Could you check a few things on this model? Use its own coordinates, in mm. Face numbers are marked on the shaded views. A direction names the side the tool comes from. Round coordinates to 2 decimals unless told otherwise and drop trailing zeros. Write each loop counter-clockwise with the first axis right and the second up, starting at its lowest first coordinate (ties: lowest second). Pieces come first, ordered by that corner, then holes. Notation, with made-up numbers: (-38.75, 12.5) - (-7.75, 12.5) arc R5 ccw to (-7.75, 20.5) - close; hole circle Ø6 at (10, 6). An arc over 180 degrees is marked (long way). Put each result on its own line as item: value.
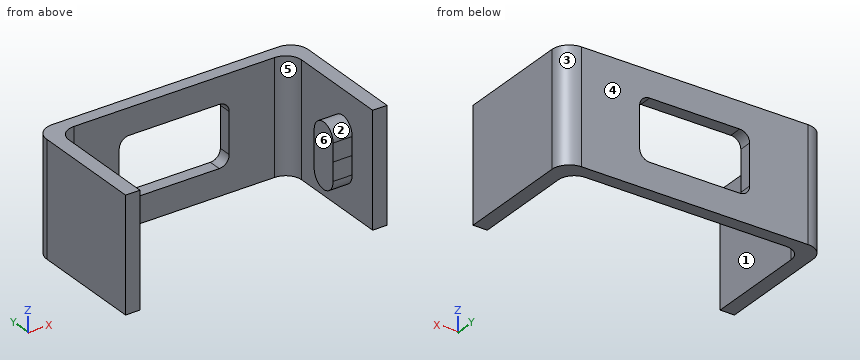
from build123d import *

# Parameters (mm, degrees)
F1_DEPTH = 9.017
F3_DEPTH = 10.288
F5_DEPTH = 2.54
F7_DEPTH = 9.017
F9_DEPTH = 25.4


with BuildPart() as f1:
    # F0 (on Top) → F1 (new body)
    with BuildSketch(Plane.XY):
        with BuildLine():
            Line((0, 9.017), (0, 0))
            Line((0, 0), (1.016, 0))
            Line((1.016, 0), (1.016, 8.128))
            ThreePointArc((1.016, 8.128), (1.387974, 9.026026), (2.286, 9.398))
            Line((2.286, 9.398), (18.288, 9.398))
            ThreePointArc((18.288, 9.398), (19.186026, 9.026026), (19.558, 8.128))
            Line((19.558, 8.128), (19.558, 0))
            Line((19.558, 0), (20.574, 0))
            Line((20.574, 0), (20.574, 9.017))
            ThreePointArc((20.574, 9.017), (20.202026, 9.915026), (19.304, 10.287))
            Line((19.304, 10.287), (1.27, 10.287))
            ThreePointArc((1.27, 10.287), (0.371974, 9.915026), (0, 9.017))
        make_face()
    extrude(amount=F1_DEPTH)

    # F2 (on face) → F3 (cut, through all)
    with BuildSketch(Plane(origin=(0, 10.287, 0), x_dir=(-1, 0, 0), z_dir=(0, 1, 0))):
        with BuildLine():
            Line((-13.87475, 2.0955), (-6.69925, 2.0955))
            ThreePointArc((-6.69925, 2.0955), (-6.137984, 2.327984), (-5.9055, 2.88925))
            Line((-5.9055, 2.88925), (-5.9055, 6.12775))
            ThreePointArc((-5.9055, 6.12775), (-6.137984, 6.689016), (-6.69925, 6.9215))
            Line((-6.69925, 6.9215), (-13.87475, 6.9215))
            ThreePointArc((-13.87475, 6.9215), (-14.436016, 6.689016), (-14.6685, 6.12775))
            Line((-14.6685, 6.12775), (-14.6685, 2.88925))
            ThreePointArc((-14.6685, 2.88925), (-14.436016, 2.327984), (-13.87475, 2.0955))
        make_face()
    extrude(amount=-F3_DEPTH, mode=Mode.SUBTRACT)

    # F4 (on face) → F5 (join)
    with BuildSketch(Plane.YZ.offset(20.574)):
        with BuildLine():
            Line((4.503683, 2.984615), (4.525844, 4.5085))
            Line((4.525844, 4.5085), (4.503683, 6.032385))
            ThreePointArc((4.503683, 6.032385), (3.385713, 7.047766), (2.345612, 5.952756))
            Line((2.345612, 5.952756), (2.366616, 4.5085))
            Line((2.366616, 4.5085), (2.345612, 3.064244))
            ThreePointArc((2.345612, 3.064244), (3.385713, 1.969234), (4.503683, 2.984615))
        make_face()
    extrude(amount=-F5_DEPTH)

    # F6 (on face) → F7 (join, through all)
    with BuildSketch(Plane(origin=(0, 0, 0), x_dir=(1, 0, 0), z_dir=(0, 0, -1))):
        with BuildLine():
            Line((20.574, 0), (20.574, -9.017))
            ThreePointArc((20.574, -9.017), (20.202026, -9.915026), (19.304, -10.287))
            Line((19.304, -10.287), (1.27, -10.287))
            ThreePointArc((1.27, -10.287), (0.371974, -9.915026), (0, -9.017))
            Line((0, -9.017), (0, 0))
            Line((0, 0), (-0.127, 0))
            Line((-0.127, 0), (-0.127, -9.017))
            ThreePointArc((-0.127, -9.017), (0.282172, -10.004828), (1.27, -10.414))
            Line((1.27, -10.414), (19.304, -10.414))
            ThreePointArc((19.304, -10.414), (20.291828, -10.004828), (20.701, -9.017))
            Line((20.701, -9.017), (20.701, 0))
            Line((20.701, 0), (20.574, 0))
        make_face()
    extrude(amount=-F7_DEPTH)

    # F8 (on face) → F9 (cut)
    with BuildSketch(Plane.XZ.offset(-10.287)):
        with BuildLine():
            ThreePointArc((5.9055, 2.88925), (6.137984, 2.327984), (6.69925, 2.0955))
            Line((6.69925, 2.0955), (13.87475, 2.0955))
            ThreePointArc((13.87475, 2.0955), (14.436016, 2.327984), (14.6685, 2.88925))
            Line((14.6685, 2.88925), (14.6685, 6.12775))
            ThreePointArc((14.6685, 6.12775), (14.436016, 6.689016), (13.87475, 6.9215))
            Line((13.87475, 6.9215), (6.69925, 6.9215))
            ThreePointArc((6.69925, 6.9215), (6.137984, 6.689016), (5.9055, 6.12775))
            Line((5.9055, 6.12775), (5.9055, 2.88925))
        make_face()
    extrude(amount=-F9_DEPTH, mode=Mode.SUBTRACT)


solid = f1.part
(1) If we mould it in two halves opening along Y, with no side actions, what happens to the marked faces 1, 2 and 3? For each: pulls with the +Y half, pulls with the -Y half, needs draft (parallel to the pull), parting line crosses it, or undercut.
Values found:
face 1: needs draft
face 2: undercut
face 3: pulls with the +Y half
(2) Imagine slicing it at B-B, the plane x = 13.5. List the corners of the cut face in (y, z) for me.
Values found:
outline: (9.4, 0) - (10.41, 0) - (10.41, 2.1) - (9.4, 2.1) - close; (9.4, 6.92) - (10.41, 6.92) - (10.41, 9.02) - (9.4, 9.02) - close
(3) Imagine slicing it at C-C, the plane z = 5.5. List the corners of the cut face in (x, y) for me, then the cut area to 3 significant figures.
Values found:
outline: (-0.13, 0) - (1.02, 0) - (1.02, 8.13) arc R1.27 cw to (2.29, 9.4) - (5.91, 9.4) - (5.91, 10.41) - (1.27, 10.41) arc R1.4 ccw to (-0.13, 9.02) - close; (14.67, 9.4) - (18.29, 9.4) arc R1.27 cw to (19.56, 8.13) - (19.56, 4.51) - (18.03, 4.51) - (18.03, 2.35) - (19.56, 2.35) - (19.56, 0) - (20.7, 0) - (20.7, 9.02) arc R1.4 ccw to (19.3, 10.41) - (14.67, 10.41) - close
area: 36.9 mm^2
(4) Imagine slicing it at A-A, the plane y = 7. List the corners of the cut face in (x, z) for me.
Values found:
outline: (-0.13, 0) - (1.02, 0) - (1.02, 9.02) - (-0.13, 9.02) - close; (19.56, 0) - (20.7, 0) - (20.7, 9.02) - (19.56, 9.02) - close
(5) For the marked faces 4, 5 and 6, which set-ups out of +Z, -Z, +X, -X, +Y, -Y let a thin tool reach every point of the face, with its end or its side?
Values found:
face 4: +Z, -Z, +X, -X, +Y
face 5: +Z, -Z
face 6: +Z, -Z, -Y
(6) I'm going to push flat-ended pins straight in: pin 1 (1.1 mm diameter, centred on y = 10, z = 4, fed in from -X); pin 2 (1.1 mm diameter, centred on y = 10, z = 4.5, fed in from +X). Where does each tip first touch, or does it pass through?
Values found:
pin 1: stops at x = -0.06
pin 2: stops at x = 20.63
(7) Please list where these lines run through material, in increasing order: probe 1 along X at (y, z) = (5.25, 4); probe 2 along X at (y, z) = (4, 3.25); probe 3 along Y at (x, z) = (17, 4.5). Write a range as from..to.
Values found:
probe 1: x = -0.13..1.02, 19.56..20.7
probe 2: x = -0.13..1.02, 18.03..20.7
probe 3: y = 9.4..10.41
(8) Imagine slicing it at D-D, the plane z = 7.5. List the corners of the cut face in (x, y) for me, then the cut area to 3 significant figures.
Values found:
outline: (-0.13, 0) - (1.02, 0) - (1.02, 8.13) arc R1.27 cw to (2.29, 9.4) - (18.29, 9.4) arc R1.27 cw to (19.56, 8.13) - (19.56, 0) - (20.7, 0) - (20.7, 9.02) arc R1.4 ccw to (19.3, 10.41) - (1.27, 10.41) arc R1.4 ccw to (-0.13, 9.02) - close
area: 42.5 mm^2
